Can you work these out from the model? Positions are in its coordinate system, mm. Face numbers are marked on the shaded views. A direction names the side the tool comes from. Give positions to 0.01 mm unless a question says otherwise; leave off trailing zeros. Write each loop counter-clockwise with the first axis right and the second up, starting at its lowest first coordinate (ties: lowest second). Pieces come first, ordered by that corner, then holes.
1. Suppose I cut it at C-C (z = 7). Please give me the cut outline in (x, y).
2. If I drill on probe 1 along Y at (x, z) = (12.5, 9); probe 2 along X at (y, z) = (-4, 13.5); probe 3 along Z at (x, y) = (6, -13), over which ranges is the centre line in solid material (lowest first)?
3. Suppose I cut it at D-D (x = -8). Please give me the cut outline in (y, z), and give its area (3 significant figures).
4. On a 3-axis mill with a long thin cutter (end or side, diameter ignored), from which of +Z, -Z, +X, -X, +Y, -Y can I reach the whole of each face in a straight line? I mean the marked faces 1, 2, 3 and 4. Say none if no direction works.
5. Suppose I cut it at A-A (z = 0). Please give me the cut outline in (x, y), and give its area (3 significant figures).
6. Thinking about a two-plate mould opening in Z: for the marked faces 5, 6 and 7, which applies, pulls with the +Z half, pulls with the -Z half, needs draft (parallel to the pull), parting line crosses it, or undercut?
7. I'm going to push flat-ended pins straight in: pin 1 (1.5 mm diameter, centred on x = 5, z = 5.5, fed in from -Y); pin 2 (12 mm diameter, centred on x = 11.5, z = -7.5, fed in from +Y). Where does each tip first touch, or does it pass through?
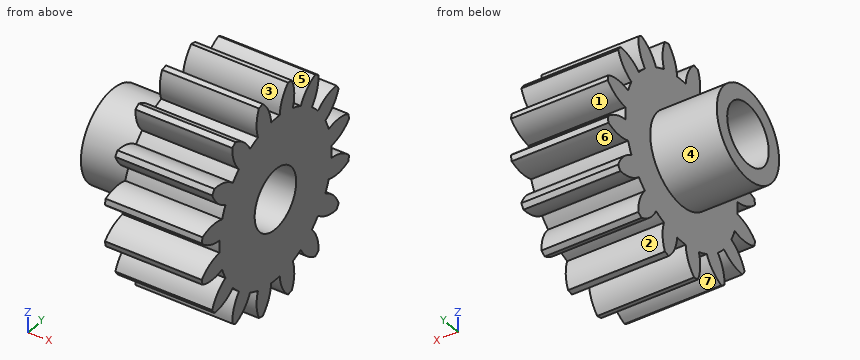
```python
from build123d import *

# Parameters (mm, degrees)
BASPROSKE_W        = 16
BASPROSKE_H        = 18
TOOTHCUT_DEPTH     = 31.066592757
TEETHCUTS_COUNT    = 16
TEETHCUTS_ANGLE    = 337.5
HUBNEAONESKE_R     = 7.5
HUBNEARONE_DEPTH   = 22.0000508
BORSKE_R           = 5
BORE_DEPTH         = 38.0000508
CUT_EXTRUDE1_START = -11
SKETCH1_R          = 7.5
CUT_EXTRUDE1_DEPTH = 11


with BuildPart() as part:
    # BasProSke → Base-Revolve (revolve)
    with BuildSketch(Plane(origin=(0, 0, 0), x_dir=(1, 0, 0), z_dir=(0, 1, 0)), mode=Mode.PRIVATE) as base_revolve_sk:
        with Locations((8, 9)):
            Rectangle(BASPROSKE_W, BASPROSKE_H)
    revolve(base_revolve_sk.sketch.rotate(Axis((-10, 0, 0), (1, 0, 0)), 180), axis=Axis((-10, 0, 0), (1, 0, 0)))

    # TooCutSke → ToothCut (cut, through all)
    with BuildSketch(Plane(origin=(0, 0, 0), x_dir=(0, 0, -1), z_dir=(1, 0, 0))):
        with BuildLine():
            ThreePointArc((1.03434411, 13.459313997), (0, 13.499), (-1.03434411, 13.459313997))
            ThreePointArc((-1.03434411, 13.459313997), (-1.635143665, 15.806872195), (-3.065655864, 17.762792553))
            ThreePointArc((-3.065655864, 17.762792553), (0, 18.0254), (3.065655864, 17.762792553))
            ThreePointArc((3.065655864, 17.762792553), (1.635143665, 15.806872195), (1.03434411, 13.459313997))
        make_face()
    toothcut = extrude(amount=TOOTHCUT_DEPTH, mode=Mode.SUBTRACT)

    # TeethCuts: ToothCut ×16 about axis
    teethcuts_axis = Axis((-10, 0, 0), (1, 0, 0))
    for i in range(1, TEETHCUTS_COUNT):
        add(toothcut.rotate(teethcuts_axis, i * TEETHCUTS_ANGLE / (TEETHCUTS_COUNT - 1)), mode=Mode.SUBTRACT)

    # HubNeaOneSke → HubNearOne (add)
    with BuildSketch(Plane.ZY):
        with Locations(Location((0, 0, 0), (0, 0, 180))):
            Circle(HUBNEAONESKE_R)
    extrude(amount=HUBNEARONE_DEPTH)

    # BorSke → Bore (cut, symmetric)
    with BuildSketch(Plane(origin=(0, 0, 0), x_dir=(0, 0, -1), z_dir=(1, 0, 0))):
        with Locations(Location((0, 0, 0), (0, 0, 180))):
            Circle(BORSKE_R)
    extrude(amount=BORE_DEPTH, both=True, mode=Mode.SUBTRACT)

    # Sketch1 → Cut-Extrude1 (cut)
    with BuildSketch(Plane.ZY.offset(22.0000508).offset(CUT_EXTRUDE1_START)):
        with Locations(Location((0, 0, 0), (0, 0, 180))):
            Circle(SKETCH1_R)
    extrude(amount=CUT_EXTRUDE1_DEPTH, mode=Mode.SUBTRACT)


solid = part.part
```
Checks:
1. outline: (-11, -2.69) - (0, -2.69) - (0, -13.4) - (16, -13.4) - (16, 13.4) - (0, 13.4) - (0, 2.69) - (-11, 2.69) - close
2. probe 1: y = -14.96 to -10.5, -10.06 to 10.06, 10.5 to 14.96
2. probe 2: x = 0 to 16
2. probe 3: z = -10.22 to -6.68, -4.25 to 4.25, 6.68 to 10.22
3. outline: circle Ø15 at (0, 0); hole circle Ø10 at (0, 0)
3. area: 98.2 mm2
4. face 1: +X, -X, +Y
4. face 2: +X, -X
4. face 3: +Z, +X, -X
4. face 4: -X
5. outline: (-11, -7.5) - (0, -7.5) - (0, -13.5) - (16, -13.5) - (16, -5) - (-11, -5) - close; (-11, 5) - (16, 5) - (16, 13.5) - (0, 13.5) - (0, 7.5) - (-11, 7.5) - close
5. area: 327 mm2
6. face 5: pulls with the +Z half
6. face 6: undercut
6. face 7: pulls with the -Z half
7. pin 1: stops at y = -12.64
7. pin 2: stops at y = 17.74
